from build123d import *
from OCP.BRepFilletAPI import BRepFilletAPI_MakeChamfer

# Parameters (mm, degrees)
SKETCH1_W           = 130
SKETCH1_H           = 7.184063047
EXTRUDE2_DEPTH      = 157
EXTRUDE3_DEPTH      = 10
EXTRUDE4_DEPTH      = 4
EXTRUDE4_DEPTH_BACK = 13
SKETCH3_R           = 38
SKETCH4_R           = 25
CUT_EXTRUDE1_DEPTH  = 173.073458762
SKETCH5_R           = 27.5
CUT_EXTRUDE2_DEPTH  = 13
CIRPATTERN1_COUNT   = 4
EXTRUDE6_DEPTH      = 10
EXTRUDE7_DEPTH      = 5
EXTRUDE7_DEPTH_BACK = 15
SKETCH11_R          = 24
SKETCH12_R          = 14
CUT_EXTRUDE3_DEPTH  = 35
CHAMFER1_SIZE       = 3
CHAMFER2_SIZE       = 3
CHAMFER3_SIZE       = 2
CHAMFER3_SIZE2      = 2.488491183
CHAMFER3_SIZE2_2    = 2.488422509
CHAMFER4_SIZE       = 3
CHAMFER4_SIZE2      = 3.751681885
SKETCH13_R          = 14.75
CUT_EXTRUDE4_DEPTH  = 1.3
FILLET3_R           = 3
SKETCH14_R          = 17.5
SKETCH14_R_2        = 11
EXTRUDE8_DEPTH      = 3.5
CIRPATTERN2_COUNT   = 4
CHAMFER8_SIZE       = 2


with BuildPart() as part:
    # Sketch1 → Extrude2 (new body)
    with BuildSketch(Plane.XY):
        with Locations((0, -70.592031523)):
            Rectangle(SKETCH1_W, SKETCH1_H)
    extrude(amount=-EXTRUDE2_DEPTH)

    # Sketch2 → Extrude3 (add)
    with BuildSketch(Plane.XY.offset(-20)):
        with BuildLine():
            Line((-60, -67), (-45.86440041, 10.269214916))
            ThreePointArc((-45.86440041, 10.269214916), (-0.018855522, 46.999996218), (45.856146013, 10.30601149))
            Line((45.856146013, 10.30601149), (60, -67))
            Line((60, -67), (-60, -67))
        make_face()
    extrude(amount=-EXTRUDE3_DEPTH)

    # Sketch3 → Extrude4 (add, two sides: drawn at the far end of the back side and taken through both)
    with BuildSketch(Plane.XY.offset(-20).offset(-EXTRUDE4_DEPTH_BACK)):
        Circle(SKETCH3_R)
    extrude(amount=EXTRUDE4_DEPTH + EXTRUDE4_DEPTH_BACK)

    # Sketch4 → Cut-Extrude1 (cut, through all)
    with BuildSketch(Plane.XY.offset(-16)):
        Circle(SKETCH4_R)
    extrude(amount=-CUT_EXTRUDE1_DEPTH, mode=Mode.SUBTRACT)

    # Sketch5 → Cut-Extrude2 (cut)
    with BuildSketch(Plane.XY.offset(-16)):
        Circle(SKETCH5_R)
    extrude(amount=-CUT_EXTRUDE2_DEPTH, mode=Mode.SUBTRACT)

    # Sketch8 → M5 Tapped Hole1 (revolve, cut)
    with BuildSketch(Plane(origin=(-0.013038394, 32.5, -16), x_dir=(0, -1, 0), z_dir=(1, 0, 0))):
        Polygon((0, 0), (0, 15.6618073), (2.1, 14.4), (2.1, 0), align=None)
    m5_tapped_hole1 = revolve(axis=Axis((-0.013038394, 32.5, -9.65), (0, 0, -1)), mode=Mode.SUBTRACT)

    # CirPattern1: M5 Tapped Hole1 ×4 about axis
    cirpattern1_axis = Axis((0, 0, 0), (0, 0, 1))
    for i in range(1, CIRPATTERN1_COUNT):
        add(m5_tapped_hole1.rotate(cirpattern1_axis, i * 360 / CIRPATTERN1_COUNT), mode=Mode.SUBTRACT)

    # Sketch10 → Extrude6 (add)
    with BuildSketch(Plane.XY.offset(-127.5)):
        with BuildLine():
            Line((-42, -67), (-28.508126396, 5.318526994))
            ThreePointArc((-28.508126396, 5.318526994), (0, 29), (28.508126396, 5.318526994))
            Line((28.508126396, 5.318526994), (42, -67))
            Line((42, -67), (-42, -67))
        make_face()
    extrude(amount=-EXTRUDE6_DEPTH)

    # Sketch11 → Extrude7 (add, two sides: drawn at the far end of the back side and taken through both)
    with BuildSketch(Plane.XY.offset(-127.5).offset(-EXTRUDE7_DEPTH_BACK)):
        Circle(SKETCH11_R)
    extrude(amount=EXTRUDE7_DEPTH + EXTRUDE7_DEPTH_BACK)

    # Sketch12 → Cut-Extrude3 (cut)
    with BuildSketch(Plane.XY.offset(-122.5)):
        Circle(SKETCH12_R)
    extrude(amount=-CUT_EXTRUDE3_DEPTH, mode=Mode.SUBTRACT)

    # Chamfer1
    chamfer1_edges = [part.edges().sort_by_distance(p)[0] for p in [
        (-38, 0, -20),
    ]]
    chamfer(chamfer1_edges, length=CHAMFER1_SIZE)

    # Chamfer2
    chamfer2_edges = [part.edges().sort_by_distance(p)[0] for p in [
        (-38, 0, -30),
    ]]
    chamfer(chamfer2_edges, length=CHAMFER2_SIZE - 0.0001)  # a hair under: the kernel refuses the full size

    # Chamfer3: one chamfer whose edges measure the first distance from different faces: ONE call of the kernel's chamfer builder (chamfer() names one face for all edges)
    chamfer3_edges_1 = [part.edges().sort_by_distance(p)[0] for p in [
        (0, -67, -30),
        (0, -67, -20),
    ]]
    chamfer3_edges_2 = [part.edges().sort_by_distance(p)[0] for p in [
        (60, -67, -25),
    ]]
    chamfer3_side_2 = [part.faces().sort_by_distance(p)[0] for p in [
        (52.928073007, -28.346994255, -25),
    ]]
    chamfer3_edges_3 = [part.edges().sort_by_distance(p)[0] for p in [
        (-60, -67, -25),
    ]]
    chamfer3_side_3 = [part.faces().sort_by_distance(p)[0] for p in [
        (0, -67, -79.525585193),
    ]]
    chamfer3 = BRepFilletAPI_MakeChamfer(part.part.solid().wrapped)
    for e in chamfer3_edges_1:
        chamfer3.Add(CHAMFER3_SIZE, e.wrapped)
    for e in chamfer3_edges_2:
        chamfer3.Add(CHAMFER3_SIZE, CHAMFER3_SIZE2, e.wrapped, chamfer3_side_2[0].wrapped)  # the first distance lies on this face
    for e in chamfer3_edges_3:
        chamfer3.Add(CHAMFER3_SIZE, CHAMFER3_SIZE2_2, e.wrapped, chamfer3_side_3[0].wrapped)  # the first distance lies on this face
    add(Compound.cast(chamfer3.Shape()), mode=Mode.REPLACE)

    # Chamfer4: one chamfer whose edges measure the first distance from different faces: ONE call of the kernel's chamfer builder (chamfer() names one face for all edges)
    chamfer4_edges_1 = [part.edges().sort_by_distance(p)[0] for p in [
        (0, -67, -137.5),
        (0, -67, -127.5),
        (-24, 0, -137.5),
        (-24, 0, -127.5),
    ]]
    chamfer4_edges_2 = [part.edges().sort_by_distance(p)[0] for p in [
        (42, -67, -132.5),
    ]]
    chamfer4_side_2 = [part.faces().sort_by_distance(p)[0] for p in [
        (35.254063198, -30.840736503, -132.5),
    ]]
    chamfer4_edges_3 = [part.edges().sort_by_distance(p)[0] for p in [
        (-42, -67, -132.5),
    ]]
    chamfer4_side_3 = [part.faces().sort_by_distance(p)[0] for p in [
        (-0.023878211, -67, -81.18589483),
    ]]
    chamfer4 = BRepFilletAPI_MakeChamfer(part.part.solid().wrapped)
    for e in chamfer4_edges_1:
        chamfer4.Add(CHAMFER4_SIZE, e.wrapped)
    for e in chamfer4_edges_2:
        chamfer4.Add(CHAMFER4_SIZE, CHAMFER4_SIZE2, e.wrapped, chamfer4_side_2[0].wrapped)  # the first distance lies on this face
    for e in chamfer4_edges_3:
        chamfer4.Add(CHAMFER4_SIZE, CHAMFER4_SIZE2, e.wrapped, chamfer4_side_3[0].wrapped)  # the first distance lies on this face
    add(Compound.cast(chamfer4.Shape()), mode=Mode.REPLACE)

    # Sketch13 → Cut-Extrude4 (cut)
    with BuildSketch(Plane.XY.offset(-126)):
        Circle(SKETCH13_R)
    extrude(amount=CUT_EXTRUDE4_DEPTH, mode=Mode.SUBTRACT)

    # Fillet3
    fillet3_edges = [part.edges().sort_by_distance(p)[0] for p in [
        (-43.5, -65.5, -139),
        (-43.5, -65.5, -126),
        (43.600744719, -65.525441738, -139.025441738),
        (43.600744719, -65.525441738, -125.974558262),
    ]]
    fillet(fillet3_edges, radius=FILLET3_R)

    # Sketch14 → Extrude8 (add)
    with BuildSketch(Plane.XY.offset(-139)):
        Circle(SKETCH14_R)
        Circle(SKETCH14_R_2, mode=Mode.SUBTRACT)
    extrude(amount=-EXTRUDE8_DEPTH)

    # Sketch15 → M5 Tapped Hole2 (revolve, cut)
    with BuildSketch(Plane(origin=(0, 18, -142.5), x_dir=(0, 1, 0), z_dir=(1, 0, 0))):
        Polygon((0, 0), (0, 16.2618073), (2.1, 15), (2.1, 0), align=None)
    m5_tapped_hole2 = revolve(axis=Axis((0, 18, -148.85), (0, 0, 1)), mode=Mode.SUBTRACT)

    # CirPattern2: M5 Tapped Hole2 ×4 about axis
    cirpattern2_axis = Axis((0, 0, 0), (0, 0, 1))
    for i in range(1, CIRPATTERN2_COUNT):
        add(m5_tapped_hole2.rotate(cirpattern2_axis, i * 360 / CIRPATTERN2_COUNT), mode=Mode.SUBTRACT)

    # Chamfer8
    chamfer8_edges = [part.edges().sort_by_distance(p)[0] for p in [
        (65, -70.592031524, -157),
        (0, -67, -157),
        (-65, -70.592031524, -157),
        (0, -67, 0),
        (65, -70.592031524, 0),
        (-65, -70.592031524, 0),
        (-65, -67, -78.5),
        (65, -67, -78.5),
    ]]
    chamfer(chamfer8_edges, length=CHAMFER8_SIZE)


solid = part.part
The model under review builds one solid part; all positions refer to its coordinate system, in mm. A direction names the side the tool comes from. Round coordinates to 2 decimals unless told otherwise and drop trailing zeros. Loops run counter-clockwise (first coordinate to the right, second up) from the corner with the lowest first, then second, coordinate; pieces in that order, holes last. Notation, with made-up numbers: (73.5, -34.5) -> (82.5, -34.5) arc R33 cw to (82.5, -0.5) -> close; hole circle Ø4 at (58, -17). An arc over 180 degrees is marked (long way). One line per question, with ' | ' between items. Start each with the question number.
Item 1: Wall thickness on line 1 along Z through (x, y) = (-32, -30); line 2 along Y through (x, z) = (-33, -13); line 3 along Z through (x, y) = (-45.5, -38): over which ranges is each line inside the solid? List them lowest first. Write a range as [from, to].
Item 2: Add section A-A, the plane z = -11. Write out the cut boundary in (x, y).
Item 3: For pin 1 (3 mm diameter, centred on x = -27, y = -25, fed in from -Z); pin 2 (5 mm diameter, centred on x = -32.5, y = -0.01, fed in from -Z); pin 3 (4 mm diameter, centred on x = -18, y = 0, fed in from -Z), all flat-tipped, find the tip position at first contact; note any pin that passes through.
Item 4: Add section B-B, the plane y = -43. Write out the cut boundary in (x, z).
Item 5: Machinability: for faces 5 (the face through (25, -8, -33)), 6 (the face through (-30.271, 23.211, -32.854)), 7 (the face through (-35, -29.48, -132.43)), 8 (the face through (12.1, -22.3, -29)), 9 (the face through (-0.09, 15.9, -135.1)), which of the approach directions +Z, -Z, +X, -X, +Y, -Y give a long, thin tool a straight path to every point of the face, cutting with its end or side? Answer none if there is none.
Item 6: Draft analysis for pull direction Y (two halves, no side actions). For faces 1 (the face through (-0.91, 46.99, -24.93)), 2 (the face through (-1, -72, 0)), 3 (the face through (-0.1, 34.6, -23.1)), 4 (the face through (17.636, 0.016, -126.457)), state which applies: +Y half, -Y half, draft (parallel to the pull), parting line (faces both ways), or undercut.
Item 7: Add section C-C, the plane x = 6. Count the separate pieces of the cut face and the enclosed holes in it, then the cut area to 3 significant figures.
Return value:
1) line 1: z = [-137.5, -127.5], [-30, -20] | line 2: y = [-74.18, -67] | line 3: z = [-30, -20]
2) outline: (-65, -74.18) -> (65, -74.18) -> (65, -69) -> (63, -67) -> (-63, -67) -> (-65, -69) -> close
3) pin 1: stops at z = -137.5 | pin 2: stops at z = -33 | pin 3: stops at z = -127.44
4) outline: (-55.61, -30) -> (55.61, -30) -> (55.61, -20) -> (-55.61, -20) -> close; (-37.52, -137.5) -> (37.52, -137.5) -> (37.52, -127.5) -> (-37.52, -127.5) -> close
5) face 5: +X, -X, +Y | face 6: none | face 7: -Z, -X, +Y | face 8: +Z | face 9: -Z
6) face 1: +Y half | face 2: draft | face 3: undercut | face 4: undercut
7) separate pieces: 3 | enclosed holes: 0 | area: 2,880 mm2
